Could you check a few things on this model? Use its own coordinates, in mm. A direction names the side the tool comes from. Coordinates: 2 decimals unless noted, no trailing zeros. Loops run counter-clockwise (first coordinate to the right, second up) from the corner with the lowest first, then second, coordinate; pieces in that order, holes last.
1) Imagine slicing it at C-C on x = 10. Please give me the cut outline in (y, z) (3 decimals), plus the area to 3 significant figures.
2) Will these pins go through, and if not, where does the flat tip stop? P1, Ø5, axis at y = 3.5, z = -14, coming from the +X side; P2, Ø1.4, axis at x = 4.5, z = -59.5, coming from the +Y side; P3, Ø3, axis at x = 3.5, y = 0.5, coming from the +Z side; P4, Ø3, axis at x = 10.5, z = -27.5, coming from the +Y side.
3) Imagine slicing it at D-D on y = 3.25. Please give me the cut outline in (x, z) (3 decimals).
4) Imagine slicing it at A-A on y = 9.75. Please give me the cut outline in (x, z) (3 decimals), plus the area to 3 significant figures.
5) For faces 5 (the face through (0, -1, -30)), 6 (the face through (6, 3, -61.595)), 7 (the face through (6, 8.128, 3)), 8 (the face through (6, 10.668, 1)), which set-ups out of +Z, -Z, +X, -X, +Y, -Y let a thin tool reach every point of the face, with its end or its side?
6) Thinking about a two-plate mould opening in Y: for faces 1 (the face through (6, 0, -29)), 2 (the face through (5.938, 12.624, 2.558)), 3 (the face through (6, 12, 3.81)), 4 (the face through (6.762, 12.624, -61.613)), which applies, released by +Y, released by -Y, zero draft, split by the parting line, or undercut?
7) Imagine slicing it at B-B on x = 6.35. Please give me the cut outline in (y, z) (3 decimals).
8) If I drill on line 1 along Z through (x, y) = (4.5, 7.5) (3 decimals); line 2 along Z through (x, y) = (3.5, 11.75) (3 decimals); line 3 along Y through (x, z) = (6.35, 2.15), over which ranges is the centre line in solid material (lowest first)?
```python
from build123d import *

# Parameters (mm, degrees)
EXTRUDE_THIN1_DEPTH       = 12.7
F_6_CLEARANCE_HOLE1_D     = 3.7973
F_6_CLEARANCE_HOLE1_DEPTH = 7.62
F_6_CLEARANCE_HOLE1_TIP   = 1.140824014
F_6_CLEARANCE_HOLE2_D     = 3.7973
F_6_CLEARANCE_HOLE2_DEPTH = 7.62
F_6_CLEARANCE_HOLE2_TIP   = 1.140824014


with BuildPart() as part:
    # Sketch1 → Extrude-Thin1 (new body)
    with BuildSketch(Plane(origin=(0, 0, 0), x_dir=(0, 0, -1), z_dir=(1, 0, 0))):
        Polygon((-1.27, 18.288), (-1.27, 10.668), (0, 10.668), (0, 0), (59.055, 0), (59.055, 10.668), (60.325, 10.668), (60.325, 18.288), (62.865, 18.288), (62.865, 8.128), (61.595, 8.128), (61.595, -2.54), (-2.54, -2.54), (-2.54, 8.128), (-3.81, 8.128), (-3.81, 18.288), align=None)
    extrude(amount=EXTRUDE_THIN1_DEPTH)

    # #6 Clearance Hole1
    with Locations(Plane(origin=(0, 0, 1.27), x_dir=(-1, 0, 0), z_dir=(0, 0, -1))):
        with Locations((-6.35, 14.478)):
            Hole(F_6_CLEARANCE_HOLE1_D / 2, depth=F_6_CLEARANCE_HOLE1_DEPTH)
            with Locations((0, 0, -(F_6_CLEARANCE_HOLE1_DEPTH + F_6_CLEARANCE_HOLE1_TIP / 2))):  # 118° drill point
                Cone(0, F_6_CLEARANCE_HOLE1_D / 2, F_6_CLEARANCE_HOLE1_TIP, mode=Mode.SUBTRACT)

    # #6 Clearance Hole2
    with Locations(Plane.XY.offset(-60.325)):
        with Locations((6.35, 14.478)):
            Hole(F_6_CLEARANCE_HOLE2_D / 2, depth=F_6_CLEARANCE_HOLE2_DEPTH)
            with Locations((0, 0, -(F_6_CLEARANCE_HOLE2_DEPTH + F_6_CLEARANCE_HOLE2_TIP / 2))):  # 118° drill point
                Cone(0, F_6_CLEARANCE_HOLE2_D / 2, F_6_CLEARANCE_HOLE2_TIP, mode=Mode.SUBTRACT)


solid = part.part
```
Filled in:
1. outline: (-2.54, -61.595) - (8.128, -61.595) - (8.128, -62.865) - (18.288, -62.865) - (18.288, -60.325) - (10.668, -60.325) - (10.668, -59.055) - (0, -59.055) - (0, 0) - (10.668, 0) - (10.668, 1.27) - (18.288, 1.27) - (18.288, 3.81) - (8.128, 3.81) - (8.128, 2.54) - (-2.54, 2.54) - close
1. area: 262 mm2
2. P1: passes through
2. P2: stops at y = 10.67
2. P3: stops at z = 2.54
2. P4: stops at y = 0
3. outline: (0, -61.595) - (12.7, -61.595) - (12.7, -59.055) - (0, -59.055) - close; (0, 0) - (12.7, 0) - (12.7, 2.54) - (0, 2.54) - close
4. outline: (0, -62.865) - (12.7, -62.865) - (12.7, -59.055) - (0, -59.055) - close; (0, 0) - (12.7, 0) - (12.7, 3.81) - (0, 3.81) - close
4. area: 96.8 mm2
5. face 5: +Z, -Z, -X, +Y, -Y
5. face 6: -Z, +X, -X, -Y
5. face 7: +Z, +X, -X, -Y
5. face 8: +X, -X, +Y
6. face 1: released by +Y
6. face 2: undercut
6. face 3: zero draft
6. face 4: undercut
7. outline: (-2.54, -61.595) - (8.128, -61.595) - (8.128, -62.865) - (12.579, -62.865) - (12.579, -60.325) - (10.668, -60.325) - (10.668, -59.055) - (0, -59.055) - (0, 0) - (10.668, 0) - (10.668, 1.27) - (12.579, 1.27) - (12.579, 3.81) - (8.128, 3.81) - (8.128, 2.54) - (-2.54, 2.54) - close; (16.377, -62.865) - (18.288, -62.865) - (18.288, -60.325) - (16.377, -60.325) - close; (16.377, 1.27) - (18.288, 1.27) - (18.288, 3.81) - (16.377, 3.81) - close
8. line 1: z = -61.595 to -59.055, 0 to 2.54
8. line 2: z = -62.865 to -60.325, 1.27 to 3.81
8. line 3: y = -2.54 to 12.58, 16.38 to 18.29
